Here's the drawing with two shaded views (mm, measured from the low corner). I have some questions. A direction names the side the tool comes from. Give positions to 0.01 mm unless a question says otherwise; leave off trailing zeros. Loops run counter-clockwise (first coordinate to the right, second up) from the corner with the lowest first, then second, coordinate; pieces in that order, holes last. Notation, with made-up numbers: (1, 18.25) -> (41, 18.25) arc R13 cw to (41, 31.25) -> close; hole circle Ø11 at (13, 75.25). An arc over 180 degrees is marked (long way). Write each question's results on one line, items separated by ' | '. Start each with the question number.
Q1. Will these pins go through, and if not, where does the flat tip stop? P1, Ø10, axis at x = 21.5, z = 19.5, coming from the +Y side; P2, Ø2, axis at x = 24.5, z = 6, coming from the +Y side; P3, Ø1, axis at x = 4, z = 22.5, coming from the +Y side.
Q2. If we section it at B-B, the plane y = 42.5: List the corners of the cut face in (x, z) for me, plus the area to 3 significant figures.
Q3. If I drill on line 1 along Z through (x, y) = (3.25, 48); line 2 along X through (y, z) = (40, 22.25); line 3 along Y through (x, z) = (15, 5.75), over which ranges is the centre line in solid material (lowest first)?
Q4. If we section it at A-A, the plane x = 15: Give the number of separate pieces and of enclosed holes in the cut face, plus the area to 3 significant figures.
Q5. We'd pull the mould along X, two halves only. Please class the marked faces 1, 2 and 3: released by +X, released by -X, zero draft, split by the parting line, or undercut.
Q6. If we section it at D-D, the plane y = 35: List the corners of the cut face in (x, z) for me, plus the area to 3 significant figures.
Q7. Which directions (+Z, -Z, +X, -X, +Y, -Y) give clear straight access to the entire face, cutting with the end or side of a thin tool? Please do the marked faces 4 and 5.
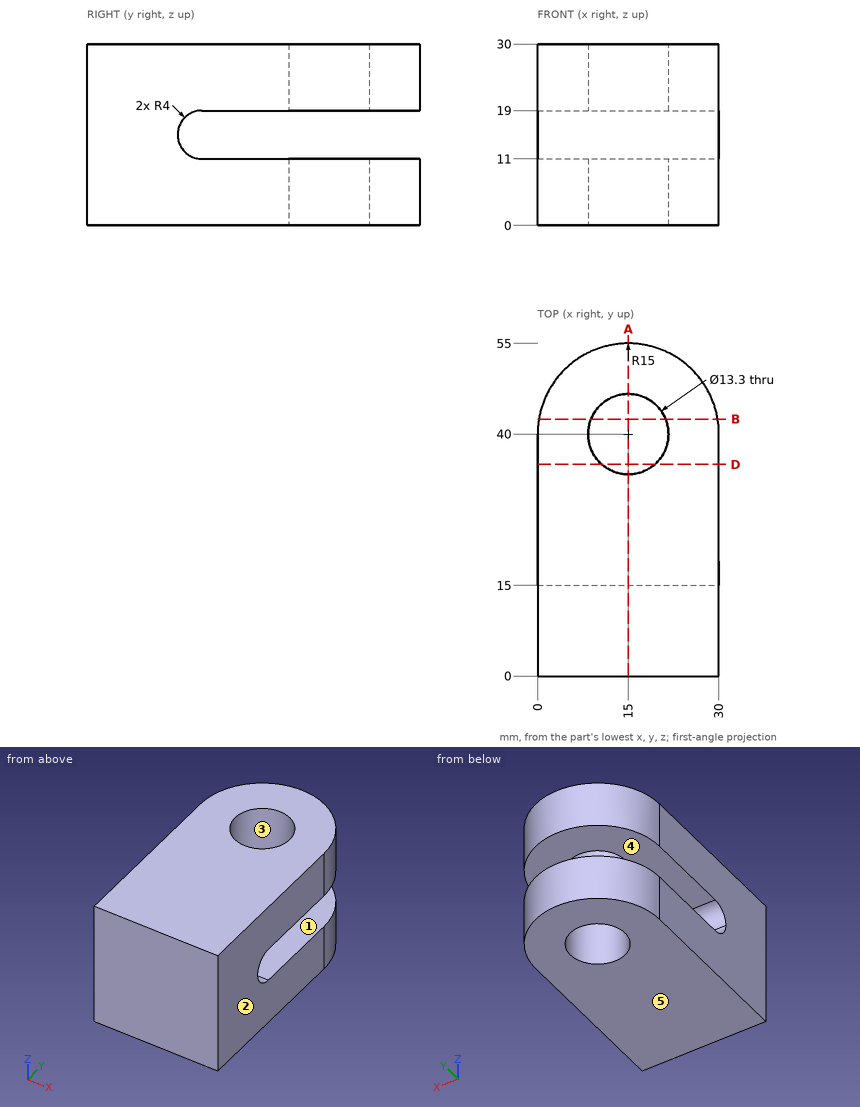
Final values:
1) P1: stops at y = 54.92 | P2: stops at y = 52.36 | P3: stops at y = 50.71
2) outline: (0.21, 0) -> (8.84, 0) -> (8.84, 11) -> (0.21, 11) -> close; (0.21, 19) -> (8.84, 19) -> (8.84, 30) -> (0.21, 30) -> close; (21.16, 0) -> (29.79, 0) -> (29.79, 11) -> (21.16, 11) -> close; (21.16, 19) -> (29.79, 19) -> (29.79, 30) -> (21.16, 30) -> close | area: 380 mm²
3) line 1: z = 0 to 11, 19 to 30 | line 2: x = 0 to 8.35, 21.65 to 30 | line 3: y = 0 to 33.35, 46.65 to 55
4) separate pieces: 3 | enclosed holes: 0 | area: 1,040 mm²
5) face 1: zero draft | face 2: released by +X | face 3: undercut
6) outline: (0, 0) -> (10.62, 0) -> (10.62, 11) -> (0, 11) -> close; (0, 19) -> (10.62, 19) -> (10.62, 30) -> (0, 30) -> close; (19.38, 0) -> (30, 0) -> (30, 11) -> (19.38, 11) -> close; (19.38, 19) -> (30, 19) -> (30, 30) -> (19.38, 30) -> close | area: 467 mm²
7) face 4: +X, -X, +Y | face 5: -Z, +X, -X, +Y, -Y
